from build123d import *

# Parameters (mm, degrees)
SKETCH_3_W               = 54
SKETCH_3_H               = 54
CUT_EXTRUDE_1_DEPTH      = 54
CUT_EXTRUDE_1_DEPTH_BACK = 54


with BuildPart() as part:
    # Sketch 1 → Revolve 1 (revolve)
    with BuildSketch(Plane.XY):
        Polygon((0, 0), (0, 13.5), (2.7, 16.2), (8.3, 16.2), (11, 13.5), (11, 0), align=None)
    revolve(axis=Axis((11, 0, 0), (-1, 0, 0)))

    # Sketch 2 → Cut-Revolve 1 (revolve, cut)
    with BuildSketch(Plane.XY):
        Polygon((0, 0), (0, 9), (0.812, 8.188), (10.188, 8.188), (11, 9), (11, 0), align=None)
    revolve(axis=Axis((11, 0, 0), (-1, 0, 0)), mode=Mode.SUBTRACT)

    # Sketch 3 → Cut-Extrude 1 (cut, two sides)
    with BuildSketch(Plane(origin=(0, 0, 0), x_dir=(0, 0, -1), z_dir=(1, 0, 0))) as cut_extrude_1_sk:
        Rectangle(SKETCH_3_W, SKETCH_3_H)
        Polygon((-13.5, -7.794228634), (0, -15.588457268), (13.5, -7.794228634), (13.5, 7.794228634), (0, 15.588457268), (-13.5, 7.794228634), align=None, mode=Mode.SUBTRACT)
    extrude(amount=CUT_EXTRUDE_1_DEPTH, mode=Mode.SUBTRACT)
    extrude(cut_extrude_1_sk.sketch, amount=-CUT_EXTRUDE_1_DEPTH_BACK, mode=Mode.SUBTRACT)


solid = part.part
For this review, take the finished solid that the model builds, in its own axes (mm). Give positions to 0.01 mm unless a question says otherwise; leave off trailing zeros. Order: outer loops, then holes, each group sorted by start corner. A loop starts at its lowest first (then second) coordinate and runs counter-clockwise, first axis right, second up. Notation, with made-up numbers: M 79.5,33.25 L 126.5,33.25 A20 cw 126.5,65.25 Z; hole C 8.5,64 d4. An arc over 180 degrees is marked long. Answer in a Markdown table with one row per item. Add a question column.
(1) For pin 1 (3 mm diameter, centred on x = 7.5, y = 10, fed in from -Z); pin 2 (1 mm diameter, centred on x = 3, y = 12, fed in from +Z), all flat-tipped, find the tip position at first contact; note any pin that passes through.
(2) Mouldability with a two-part tool opening along Z and no side actions: class faces 1 (the face through (11, 9, 3)), 2 (the face through (5, 0, -13.5)), 3 (the face through (5.566, -1.775, 7.993)) as +Z half, -Z half, draft (parallel to the pull), parting line (faces both ways), or undercut.
(3) Consider section A-A on x = 5. State the section outline as (y, z) points.
(4) Wall thickness on probe 1 along Z at (x, y) = (1.25, -2); probe 2 along Z at (x, y) = (4, 6); probe 3 along Y at (x, z) = (2.25, -2.5): over which ranges is each line inside the solid? List them lowest first. Write a range as [from, to].
Evaluation:
| question | item | result |
|---|---|---|
| 1 | pin 1 | stops at z = -12.28 |
| 1 | pin 2 | stops at z = 7.08 |
| 2 | face 1 | draft |
| 2 | face 2 | -Z half |
| 2 | face 3 | undercut |
| 3 | outline | M -15.59,0 L -7.79,-13.5 L 7.79,-13.5 L 15.59,0 L 7.79,13.5 L -7.79,13.5 Z; hole C 0,0 d16.38 |
| 4 | probe 1 | z = [-13.5, -7.94], [7.94, 13.5] |
| 4 | probe 2 | z = [-13.5, -5.57], [5.57, 13.5] |
| 4 | probe 3 | y = [-14.15, -7.8], [7.8, 14.15] |
